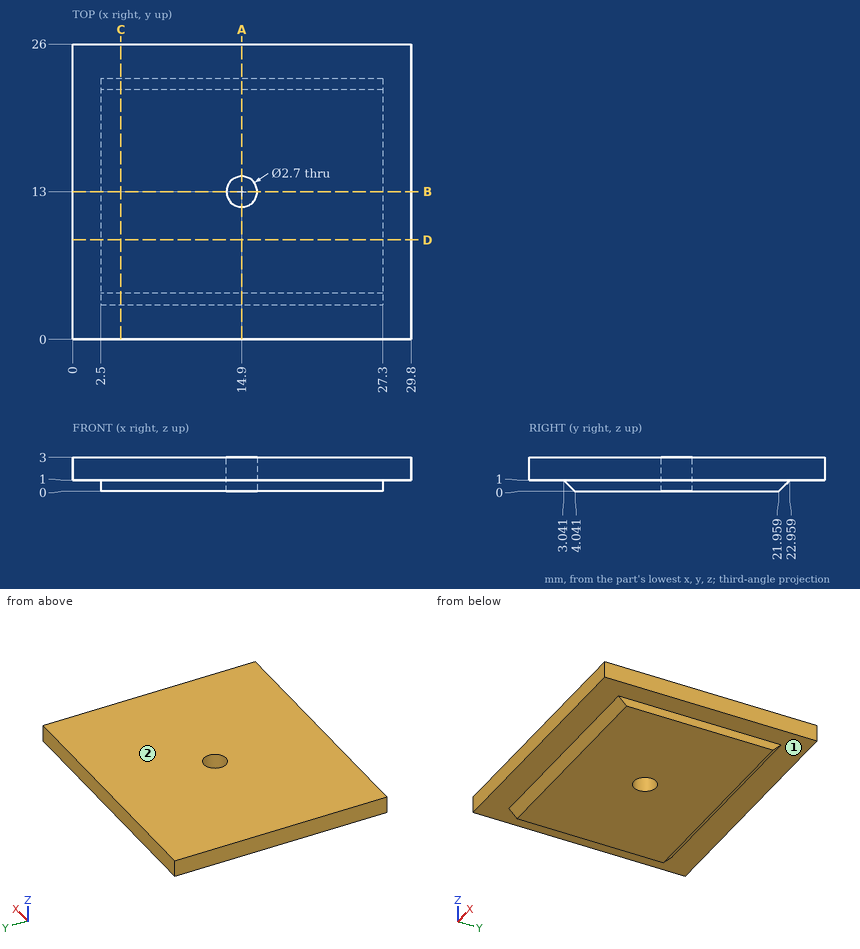
Verification items for this drawing (mm, ordinates from the low corner). A direction names the side the tool comes from. Give positions to 0.01 mm unless a question says otherwise; leave off trailing zeros. Write each loop counter-clockwise with the first axis right and the second up, starting at its lowest first coordinate (ties: lowest second). Pieces come first, ordered by that corner, then holes. Notation, with made-up numbers: (-26.75, -11) -> (31.25, -11) arc R18 cw to (31.25, 6) -> close; hole circle Ø5 at (16.25, 72). An arc over 180 degrees is marked (long way). Use CSV: the item, a comma, the result in double quotes. Start each with the question number.
Q1. Tool access check on the marked faces 1 and 2. Record the directions out of +Z, -Z, +X, -X, +Y, -Y that give a thin tool (end or side, any length) a straight path to the whole face; none if there is none.
Q2. Depth check by flat-ended pin: P1, Ø0.5, axis at y = 11.5, z = 0.5, coming from the +X side. Enter the tip coordinate at first touch or a pass-through.
Q3. Scan lines: line 1 along Y through (x, z) = (14.9, 1.9); line 2 along X through (y, z) = (13.75, 1.05); line 3 along Z through (x, y) = (28.75, 1.5). Record each from-to range of solid material in increasing order.
Q4. Cross-section at B-B on y = 13. Enter the section's corners in (x, z).
Q5. Cross-section at A-A on x = 14.9. Enter the section's corners in (y, z).
Q6. Cross-section at C-C on x = 4.25. Enter the section's corners in (y, z).
Q7. Cross-section at D-D on y = 8.75. Enter the section's corners in (x, z).
Working result:
1,face 1,"-Z"
1,face 2,"+Z, +X, -X, +Y, -Y"
2,P1,"stops at x = 27.3"
3,line 1,"y = 0 to 11.65, 14.35 to 26"
3,line 2,"x = 0 to 13.78, 16.02 to 29.8"
3,line 3,"z = 1 to 3"
4,outline,"(0, 1) -> (2.5, 1) -> (2.5, 0) -> (13.55, 0) -> (13.55, 3) -> (0, 3) -> close; (16.25, 0) -> (27.3, 0) -> (27.3, 1) -> (29.8, 1) -> (29.8, 3) -> (16.25, 3) -> close"
5,outline,"(0, 1) -> (3.04, 1) -> (4.04, 0) -> (11.65, 0) -> (11.65, 3) -> (0, 3) -> close; (14.35, 0) -> (21.96, 0) -> (22.96, 1) -> (26, 1) -> (26, 3) -> (14.35, 3) -> close"
6,outline,"(0, 1) -> (3.04, 1) -> (4.04, 0) -> (21.96, 0) -> (22.96, 1) -> (26, 1) -> (26, 3) -> (0, 3) -> close"
7,outline,"(0, 1) -> (2.5, 1) -> (2.5, 0) -> (27.3, 0) -> (27.3, 1) -> (29.8, 1) -> (29.8, 3) -> (0, 3) -> close"
